Geometry check sheet. Reference: the model listing, model coordinates, mm. A direction names the side the tool comes from. Give positions to 0.01 mm unless a question says otherwise; leave off trailing zeros. Loops run counter-clockwise (first coordinate to the right, second up) from the corner with the lowest first, then second, coordinate; pieces in that order, holes last. Notation, with made-up numbers: (0.5, 36.25) - (40.5, 36.25) arc R16 cw to (40.5, 65.25) - close; hole circle Ø11 at (-38, 48). An arc over 180 degrees is marked (long way). Write item = value, one per line. Start each with the question number.
from build123d import *

# Parameters (mm, degrees)
F0_W      = 55
F0_H      = 19
F1_DEPTH  = 26
F2_W      = 55
F2_H      = 14
F3_DEPTH  = 25
F4_W      = 19
F4_H      = 12
F5_DEPTH  = 10
F6_W      = 19
F6_H      = 12
F7_DEPTH  = 10
F8_R      = 1.85
F9_DEPTH  = 44
F10_DEPTH = 44
F11_R     = 2.25
F11_R_2   = 2.2993583235
F12_DEPTH = 12
F13_W     = 10
F13_H     = 5.5
F14_DEPTH = 5


with BuildPart() as f1:
    # F0 (on Top) → F1 (new body)
    with BuildSketch(Plane.XY):
        Rectangle(F0_W, F0_H)
    extrude(amount=F1_DEPTH)

    # F2 (on face) → F3 (join)
    with BuildSketch(Plane(origin=(0, 9.5, 0), x_dir=(-1, 0, 0), z_dir=(0, 1, 0))):
        with Locations((0, 7)):
            Rectangle(F2_W, F2_H)
    extrude(amount=F3_DEPTH)

    # F4 (on face) + F3_face1 (on face) → F5 (join)
    with BuildSketch(Plane(origin=(-27.5, 0, 0), x_dir=(0, -1, 0), z_dir=(-1, 0, 0))):
        with Locations((0, 20)):
            Rectangle(F4_W, F4_H)
    with BuildSketch(Plane(origin=(27.5, 9.1232227488, 10.5118483412), x_dir=(0, 1, 0), z_dir=(1, 0, 0))):
        Polygon((-18.6232227488, 15.4881516588), (-18.6232227488, -10.5118483412), (25.3767772512, -10.5118483412), (25.3767772512, 3.4881516588), (0.3767772512, 3.4881516588), (0.3767772512, 15.4881516588), align=None)
    extrude(amount=F5_DEPTH, dir=(-1, 0, 0))

    # F6 (on face) → F7 (join)
    with BuildSketch(Plane.YZ.offset(27.5)):
        with Locations((0, 20)):
            Rectangle(F6_W, F6_H)
    extrude(amount=F7_DEPTH)

    # F8 (on face) → F9 (cut)
    with BuildSketch(Plane(origin=(0, 34.5, 0), x_dir=(-1, 0, 0), z_dir=(0, 1, 0))):
        with Locations((-21, 7)):
            Circle(F8_R)
        with Locations((21, 7)):
            Circle(F8_R)
    extrude(amount=-F9_DEPTH, mode=Mode.SUBTRACT)

    # F8 (on face) → F10 (cut)
    with BuildSketch(Plane(origin=(0, 34.5, 0), x_dir=(-1, 0, 0), z_dir=(0, 1, 0))):
        with Locations((-21, 7)):
            Circle(F8_R)
        with Locations((21, 7)):
            Circle(F8_R)
    extrude(amount=-F10_DEPTH, mode=Mode.SUBTRACT)

    # F11 (on face) → F12 (cut)
    with BuildSketch(Plane.XY.offset(26)):
        with Locations((32.5, 0)):
            Circle(F11_R)
        with Locations((-32.5, 0)):
            Circle(F11_R_2)
    extrude(amount=-F12_DEPTH, mode=Mode.SUBTRACT)

    # F13 (on face) → F14 (join)
    with BuildSketch(Plane.XY.offset(26)):
        with Locations((17.5, 0)):
            Rectangle(F13_W, F13_H)
        with Locations((-17.5, 0)):
            Rectangle(F13_W, F13_H)
    extrude(amount=F14_DEPTH)


solid = f1.part
1) Material ranges on line 1 along Y through (x, z) = (32.5, 21); line 2 along Y through (x, z) = (-32.5, 22.75); line 3 along Z through (x, y) = (4, -5), recorded low to high.
2) Gauge pin test, flat ends, axial feed: P1, Ø6, axis at x = 11.5, z = 21.5, coming from the +Y side; P2, Ø1.5, axis at y = 27, z = 8, coming from the +X side; P3, Ø2.5, axis at y = -1, z = 27.5, coming from the -X side. Record the tip position at first contact, or that the pin passes through.
3) Tool access check on faces 5 (the face through (12.5, 0, 28)), 6 (the face through (17, -2.75, 28)), 7 (the face through (30, 0, 14)), 8 (the face through (-27.5, 12, 7)), 9 (the face through (-1, 9.5, 20)). Record the directions out of +Z, -Z, +X, -X, +Y, -Y that give a thin tool (end or side, any length) a straight path to the whole face; none if there is none.
4) Cross-section at B-B on x = -32.5. Enter the section's corners in (y, z), and give its area (3 significant figures).
5) Cross-section at C-C on z = 20. Enter the section's corners in (x, y).
6) Release check for a two-part mould opening along Y. For faces 1 (the face through (-1, 0, 26)), 2 (the face through (-30.307, 0.691, 20.084)), 3 (the face through (-1, -9.5, 13)), 4 (the face through (34.58, -0.86, 20.08)) record: pulls with the +Y half, pulls with the -Y half, needs draft (parallel to the pull), parting line crosses it, or undercut.
7) Cross-section at A-A on y = 0. Enter the section's corners in (x, z), and give its area (3 significant figures).
8) Cross-section at D-D on y = -5. Enter the section's corners in (x, z).
Checked values:
q1.line_1 = -9.5 to -2.25, 2.25 to 9.5
q1.line_2 = -9.5 to -2.3, 2.3 to 9.5
q1.line_3 = 0 to 26
q2.P1 = 9.5
q2.P2 = 27.5
q2.P3 = -22.5
q3.face_5 = +Z, +Y, -Y
q3.face_6 = +Z, +X, -X, -Y
q3.face_7 = -Z, +X, +Y, -Y
q3.face_8 = -Z, -X, +Y, -Y
q3.face_9 = +Z, +X, -X, +Y
q4.outline = (-9.5, 14) - (-2.3, 14) - (-2.3, 26) - (-9.5, 26) - close; (2.3, 14) - (9.5, 14) - (9.5, 26) - (2.3, 26) - close
q4.area = 173 mm²
q5.outline = (-37.5, -9.5) - (37.5, -9.5) - (37.5, 9.5) - (-37.5, 9.5) - close; hole circle Ø4.6 at (-32.5, 0); hole circle Ø4.5 at (32.5, 0)
q6.face_1 = needs draft
q6.face_2 = undercut
q6.face_3 = pulls with the -Y half
q6.face_4 = undercut
q7.outline = (-37.5, 14) - (-34.8, 14) - (-34.8, 26) - (-37.5, 26) - close; (-30.2, 14) - (-27.5, 14) - (-27.5, 0) - (27.5, 0) - (27.5, 14) - (30.25, 14) - (30.25, 26) - (22.5, 26) - (22.5, 31) - (12.5, 31) - (12.5, 26) - (-12.5, 26) - (-12.5, 31) - (-22.5, 31) - (-22.5, 26) - (-30.2, 26) - close; (34.75, 14) - (37.5, 14) - (37.5, 26) - (34.75, 26) - close; hole circle Ø3.7 at (-21, 7); hole circle Ø3.7 at (21, 7)
q7.area = 1,640 mm²
q8.outline = (-37.5, 14) - (-27.5, 14) - (-27.5, 0) - (27.5, 0) - (27.5, 14) - (37.5, 14) - (37.5, 26) - (-37.5, 26) - close; hole circle Ø3.7 at (-21, 7); hole circle Ø3.7 at (21, 7)
